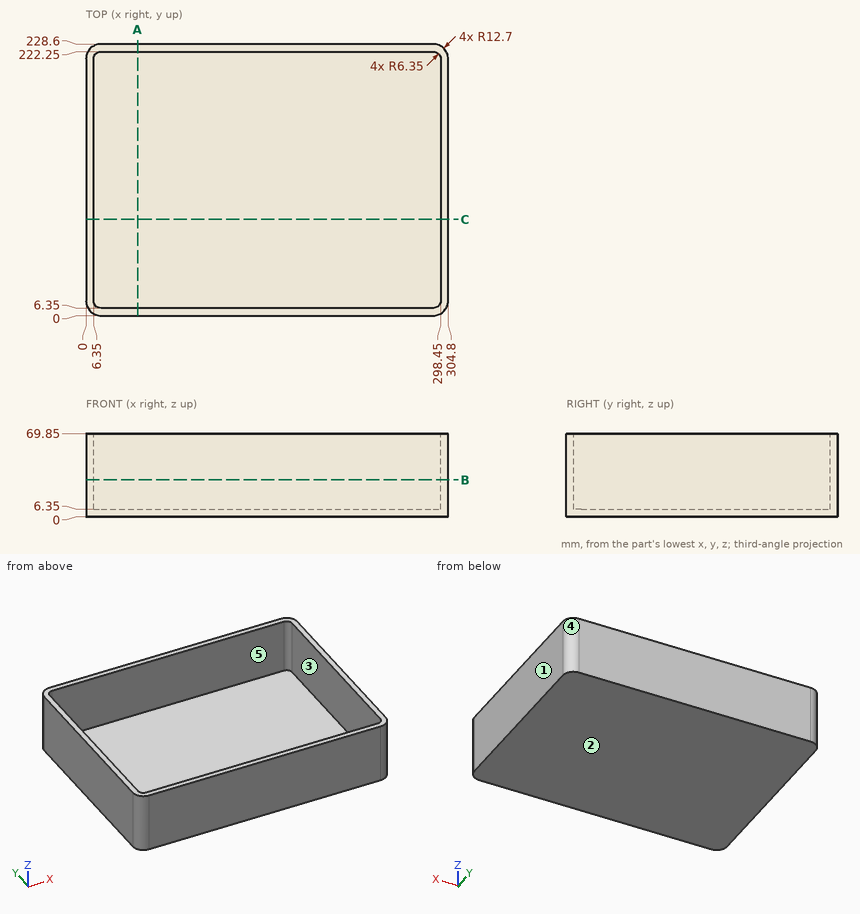
The figure shows three views and two pictorial views of one solid part (mm, origin at its lowest corner). Answer the questions. A direction names the side the tool comes from. Give positions to 0.01 mm unless a question says otherwise; leave off trailing zeros. Write each loop counter-clockwise with the first axis right and the second up, starting at its lowest first coordinate (ties: lowest second). Pieces come first, ordered by that corner, then holes. Notation, with made-up numbers: (-20.75, 40) - (14.25, 40) arc R27 ccw to (14.25, 60) - close; hole circle Ø7 at (8, -0.75). An arc over 180 degrees is marked (long way). Use CSV: the item, a comma, the result in double quotes. Start each with the question number.
Item 1: The part is cut by section C-C, the plane y = 81. Give the vertices of the cut face in (x, z), and give its area (3 significant figures).
Item 2: Consider line 1 (X direction, y = 174.5, z = 28); line 2 (Y direction, x = 97.5, z = 65); line 3 (Z direction, x = 135.5, y = 41.5). Determine where each line is inside the solid, lowest interval first.
Item 3: For the marked faces 4 and 5, determine the directions among +Z, -Z, +X, -X, +Y, -Y from which every point of the face is accessible in a straight line to the end or side of a thin tool.
Item 4: The part is cut by section A-A, the plane x = 43.5. Give the vertices of the cut face in (y, z).
Item 5: The part is cut by section B-B, the plane z = 31. Give the vertices of the cut face in (x, y), and give its area (3 significant figures).
Item 6: The mould has two halves that part along X. Classify the marked faces 1, 2 and 3: pulls with the +X half, pulls with the -X half, needs draft (parallel to the pull), parting line crosses it, or undercut.
Taken from the geometry:
1,outline,"(0, 0) - (304.8, 0) - (304.8, 69.85) - (298.45, 69.85) - (298.45, 6.35) - (6.35, 6.35) - (6.35, 69.85) - (0, 69.85) - close"
1,area,"2,740 mm2"
2,line 1,"0 to 6.35, 298.45 to 304.8"
2,line 2,"0 to 6.35, 222.25 to 228.6"
2,line 3,"0 to 6.35"
3,face 4,"+Z, -Z, +X, +Y"
3,face 5,"+Z"
4,outline,"(0, 0) - (228.6, 0) - (228.6, 69.85) - (222.25, 69.85) - (222.25, 6.35) - (6.35, 6.35) - (6.35, 69.85) - (0, 69.85) - close"
5,outline,"(0, 12.7) arc R12.7 ccw to (12.7, 0) - (292.1, 0) arc R12.7 ccw to (304.8, 12.7) - (304.8, 215.9) arc R12.7 ccw to (292.1, 228.6) - (12.7, 228.6) arc R12.7 ccw to (0, 215.9) - close; hole (6.35, 12.7) arc R6.35 ccw to (12.7, 6.35) - (292.1, 6.35) arc R6.35 ccw to (298.45, 12.7) - (298.45, 215.9) arc R6.35 ccw to (292.1, 222.25) - (12.7, 222.25) arc R6.35 ccw to (6.35, 215.9) - close"
5,area,"6,510 mm2"
6,face 1,"pulls with the +X half"
6,face 2,"needs draft"
6,face 3,"undercut"
